Build history of the part. All positions in model axes, mm. Round coordinates to 2 decimals unless told otherwise and drop trailing zeros. Write each loop counter-clockwise with the first axis right and the second up, starting at its lowest first coordinate (ties: lowest second). Pieces come first, ordered by that corner, then holes.
Autodesk Inventor part; units mm, degrees
ref_plane "YZ Plane" through (0, 0, 0) normal (1, 0, 0) x (0, 1, 0)
ref_plane "XZ Plane" through (0, 0, 0) normal (0, 1, 0) x (-1, 0, 0)
ref_plane "XY Plane" through (0, 0, 0) normal (0, 0, 1) x (1, 0, 0)
sketch "Sketch1" plane through (0, 0, 0) normal (0, 0, 1) x (1, 0, 0)
  line L0 (-1498, 0) -> (1498, 0) construction
  line L1 (-1498, 0) -> (-898, 0)
  line L2 (-898, 0) -> (-898, 2068)
  line L3 (-898, 2068) -> (-1498, 2068)
  line L4 (-1498, 2068) -> (-1498, 0)
  line L5 (-898, 0) -> (-498, 0)
  line L6 (-498, 0) -> (-498, 816)
  line L7 (-498, 816) -> (-898, 816)
  line L8 (-898, 816) -> (-898, 0)
  line L9 (-498, 0) -> (102, 0)
  line L10 (102, 0) -> (102, 816)
  line L11 (102, 816) -> (-498, 816)
  line L12 (-498, 816) -> (-498, 0)
  line L13 (102, 0) -> (698, 0)
  line L14 (698, 0) -> (698, 668)
  line L15 (698, 668) -> (102, 668)
  line L16 (102, 668) -> (102, 0)
  line L17 (698, 0) -> (1498, 0)
  line L18 (1498, 0) -> (1498, 816)
  line L19 (1498, 816) -> (698, 816)
  line L20 (698, 816) -> (698, 0)
  line L21 (-1498, 0) -> (1498, 0)
  line L22 (1498, 0) -> (1498, 96)
  line L23 (1498, 96) -> (-1498, 96)
  line L24 (-1498, 96) -> (-1498, 0)
  line L25 (-898, 816) -> (1498, 816)
  line L26 (1498, 816) -> (1498, 832)
  line L27 (1498, 832) -> (-898, 832)
  line L28 (-898, 832) -> (-898, 816)
  line L29 (-898, 1972) -> (-498, 1972)
  line L30 (-498, 1972) -> (-498, 1372)
  line L31 (-498, 1372) -> (-898, 1372)
  line L32 (-898, 1372) -> (-898, 1972)
  line L33 (698, 1972) -> (1498, 1972)
  line L34 (1498, 1972) -> (1498, 1372)
  line L35 (1498, 1372) -> (698, 1372)
  line L36 (698, 1372) -> (698, 1972)
  line L37 (698, 1372) -> (98, 1372)
  line L38 (98, 1372) -> (98, 1972)
  line L39 (98, 1972) -> (698, 1972)
  line L40 (698, 1972) -> (698, 1372)
  line L41 (-498, 1372) -> (98, 1372)
  line L42 (-498, 1372) -> (-275, 1637.7611)
  line L43 (98, 1372) -> (-125, 1637.7611)
  line L44 (-275, 1637.7611) -> (-125, 1637.7611)
  line L45 (-125, 1637.7611) -> (-125, 2068)
  line L46 (-125, 2068) -> (-275, 2068)
  line L47 (-275, 2068) -> (-275, 1637.7611)
  line L48 (1098, 816) -> (1098, 96)
  line L49 (-198, 816) -> (-198, 96)
  line L50 (-898, 668) -> (-498, 668)
  line L51 (-1498, 520) -> (-898, 520)
  line L52 (-1498, 1579) -> (-898, 1579)
  line L53 (398, 1972) -> (398, 1372)
  line L54 (1098, 1972) -> (1098, 1372)
  line L55 (698, 1876) -> (1498, 1876)
  line L56 (698, 1468) -> (1498, 1468)
  line L57 (-1498, 1049.5) -> (-898, 1049.5)
  point P0 (0, 0)
  point P1 (0, 0)
  point P2 (0, 0)
  point P3 (-198, 816)
  point P4 (0, 0)
  point P5 (102, 668)
  dimension "d0" = 2996
  dimension "d1" = 600
  dimension "d2" = 2068
  dimension "d3" = 400
  dimension "d4" = 816
  dimension "d5" = 600
  dimension "d6" = 816
  dimension "d7" = 596
  dimension "d8" = 668
  dimension "d9" = 800
  dimension "d10" = 816
  dimension "d11" = 96
  dimension "d12" = 16
  dimension "d13" = 400
  dimension "d14" = 600
  dimension "d15" = 96
  dimension "d16" = 800
  dimension "d17" = 600
  dimension "d18" = 600
  dimension "d19" = 600
  dimension "d20" = 50
  dimension "d21" = 150
  dimension "d22" = 148
  dimension "d23" = 1059
  dimension "d24" = 96
  dimension "d25" = 96
  dimension "d26" = 529.5
extrude "Extrusion1" add sketch "Sketch1" along normal blind 12 contours L10 L25 L20 L15
sketch "Sketch2" plane through (0, 0, 12) normal (0, 0, 1) x (1, 0, 0)
  line L0 (698, 816) -> (102, 816)
  line L1 (102, 816) -> (698, 816)
  line L2 (698, 816) -> (698, 813)
  line L3 (698, 813) -> (102, 813)
  line L4 (102, 813) -> (102, 816)
  point P0 (0, 0)
  dimension "d29" = 3
extrude "Extrusion2" cut sketch "Sketch2" against normal blind 67
sketch "Sketch3" plane through (0, 0, 12) normal (0, 0, 1) x (1, 0, 0)
  line L0 (225, 773) -> (575, 773)
  line L1 (575, 773) -> (575, 708)
  line L2 (575, 708) -> (225, 708)
  line L3 (225, 708) -> (225, 773)
  line L4 (698, 668) -> (698, 813)
  line L5 (698, 813) -> (102, 813)
  point P0 (0, 0)
  point P1 (575, 740.5)
  point P2 (698, 740.5)
  point P3 (400, 773)
  point P4 (400, 813)
  dimension "d32" = 65
  dimension "d33" = 350
extrude "Extrusion3" cut sketch "Sketch3" against normal blind 3
properties part number "Dummy Washing Machine"
1) Slice it at B-B (y = 734). Write the cut outline in (x, z).
Results:
outline: (102, 0) - (698, 0) - (698, 12) - (575, 12) - (575, 9) - (225, 9) - (225, 12) - (102, 12) - close
2) Wall check: L1, parallel to X at y = 763, z = 9.75; L2, parallel to Z at x = 256, y = 769; L3, parallel to Y at x = 546, z = 10.5. Give the ranges that are in metal, low to high.
Results:
L1: x = 102 to 225, 575 to 698
L2: z = 0 to 9
L3: y = 668 to 708, 773 to 813
3) Mould opens along X. For faces 1 (the flat face through (404, 813, 6)), 2 (the flat face through (398, 741, 9)), 3 (the flat face through (698, 742, 6)) say: released by +X, released by -X, zero draft, split by the parting line, or undercut.
Results:
face 1: zero draft
face 2: undercut
face 3: released by +X
4) Slice it at A-A (x = 472). Write the cut outline in (y, z).
Results:
outline: (668, 0) - (813, 0) - (813, 12) - (773, 12) - (773, 9) - (708, 9) - (708, 12) - (668, 12) - close
5) Pin check, flat tip, straight feed: pin 1 Ø12 at (x, y) = (416, 736.5) entering from +Z. Stop position of the tip, or through.
Results:
pin 1: stops at z = 9
